```python
from build123d import *

# Parameters (mm, degrees)
F0_W     = 224
F0_H     = 233
F0_R     = 2.5
F1_DEPTH = 3
F2_W     = 223.902777
F2_H     = 20.5527
F3_DEPTH = 10
F4_SIZE  = 8
F5_R     = 10
F6_R     = 10


with BuildPart() as f1:
    # F0 (on Top) → F1 (new body)
    with BuildSketch(Plane.XY):
        with Locations((-34.568664, -44.312108)):
            Rectangle(F0_W, F0_H)
        with Locations((-34.568664, 67.187892)):
            Circle(F0_R, mode=Mode.SUBTRACT)
    extrude(amount=F1_DEPTH)

    # F2 (on face) → F3 (join)
    with BuildSketch(Plane.XZ.offset(160.812108)):
        with Locations((-34.617275, 10.27635)):
            Rectangle(F2_W, F2_H)
    extrude(amount=F3_DEPTH)

    # F4
    f4_edges = [f1.edges().sort_by_distance(p)[0] for p in [
        (-34.617275, -160.812108, 20.5527),
    ]]
    chamfer(f4_edges, length=F4_SIZE)

    # F5
    f5_edges = [f1.edges().sort_by_distance(p)[0] for p in [
        (-146.568664, 72.187892, 1.5),
    ]]
    fillet(f5_edges, radius=F5_R)

    # F6
    f6_edges = [f1.edges().sort_by_distance(p)[0] for p in [
        (77.431336, 72.187892, 1.5),
    ]]
    fillet(f6_edges, radius=F6_R)


solid = f1.part
```
Check sheet for the modelled part. Datum: model origin and axes. Units: mm. A direction names the side the tool comes from. Round coordinates to 2 decimals unless told otherwise and drop trailing zeros. Order: outer loops, then holes, each group sorted by start corner. A loop starts at its lowest first (then second) coordinate and runs counter-clockwise, first axis right, second up.
1) Section check A-A (x = -79.5). Record the boundary of the cut face in (y, z), and give its area (3 significant figures).
2) Scan lines: line 1 (Y direction, x = -115.5, z = 7.25); line 2 (Z direction, x = 46.5, y = -119.5); line 3 (Y direction, x = -126.5, z = 19). Record each from-to range of solid material in increasing order.
3) Mould release check, pull along Y, two halves, no side actions. Record for faces 1 (the cylindrical face through (-32.26, 66.23, 1.48)), 2 (the flat face through (-36, -170.812, 10)), 3 (the flat face through (-36.18, -164.76, 16.5)): +Y half, -Y half, draft (parallel to the pull), parting line (faces both ways), or undercut.
4) Tool access check on faces 4 (the cylindrical face through (74.42, 69.34, 1.52)), 5 (the flat face through (-36, -43, 3)). Record the directions out of +Z, -Z, +X, -X, +Y, -Y that give a thin tool (end or side, any length) a straight path to the whole face; none if there is none.
5) Section check B-B (y = -85). Record the boundary of the cut face in (x, z).
6) Section check C-C (z = 6.75). Record the boundary of the cut face in (x, y).
7) Go/stop test with flat-tipped pins: pin 1 Ø1.5 at (x, y) = (-35.5, -145) entering from +Z; pin 2 Ø3 at (x, z) = (-11.5, 9.5) entering from +Y. Record where each tip stops, or that it passes through.
Result:
1. outline: (-170.81, 0) - (72.19, 0) - (72.19, 3) - (-160.81, 3) - (-160.81, 12.55) - (-168.81, 20.55) - (-170.81, 20.55) - close
1. area: 873 mm2
2. line 1: y = -170.81 to -160.81
2. line 2: z = 0 to 3
2. line 3: y = -170.81 to -167.26
3. face 1: undercut
3. face 2: -Y half
3. face 3: +Y half
4. face 4: +Z, -Z, +X, +Y
4. face 5: +Z, +X, -X, +Y
5. outline: (-146.57, 0) - (77.43, 0) - (77.43, 3) - (-146.57, 3) - close
6. outline: (-146.57, -170.81) - (77.33, -170.81) - (77.33, -160.81) - (-146.57, -160.81) - close
7. pin 1: stops at z = 3
7. pin 2: stops at y = -160.81
